Source: three-view drawing plus pictorial views. Frame: mm from the lowest corner of the part. A direction names the side the tool comes from. Coordinates: 2 decimals unless noted, no trailing zeros. Write each loop counter-clockwise with the first axis right and the second up, starting at its lowest first coordinate (ties: lowest second). Pieces come first, ordered by that corner, then holes. Notation, with made-up numbers: (3.25, -17) - (51.25, -17) arc R31 cw to (51.25, 21) - close; hole circle Ø10 at (28.25, -14). An arc over 180 degrees is marked (long way). Answer as a JSON object with one key per item and string values. Group by question number.
Item 1: Section A-A on x = 18. Return loops of the section in (y, z).
Item 2: Section C-C on z = 143. Return loops of the section in (x, y).
Item 3: Set-up query: the marked faces 4, 5 and 6. Return all of +Z, -Z, +X, -X, +Y, -Y with unobstructed straight access to the full face (end or side cutting, diameter ignored); none if empty.
Item 4: Mould query, pull axis Z, two halves, no side actions, for the marked faces 1, 2 and 3. Classes: pulls with the +Z half, pulls with the -Z half, needs draft (parallel to the pull), parting line crosses it, or undercut.
Item 5: First-contact query: pin 1 Ø15 at (y, z) = (128.5, 97) entering from +X; pin 2 Ø17 at (x, z) = (22, 64) entering from +Y; pin 3 Ø23 at (x, z) = (32, 120.5) entering from +Y. Flat tips, straight axial feed; report the tip coordinate or a pass-through.
Item 6: Line query: line 1 along Y through (x, z) = (71.5, 204); line 2 along Y through (x, z) = (33, 120); line 3 along Y through (x, z) = (5.5, 87.5). Output: solid intervals per line, ascending. Write a range as from..to.
Item 7: Section B-B on y = 57. Return loops of the section in (x, z), and give its area (3 significant figures).
Item 8: Section D-D on x = 51. Return loops of the section in (y, z), and give its area (3 significant figures).
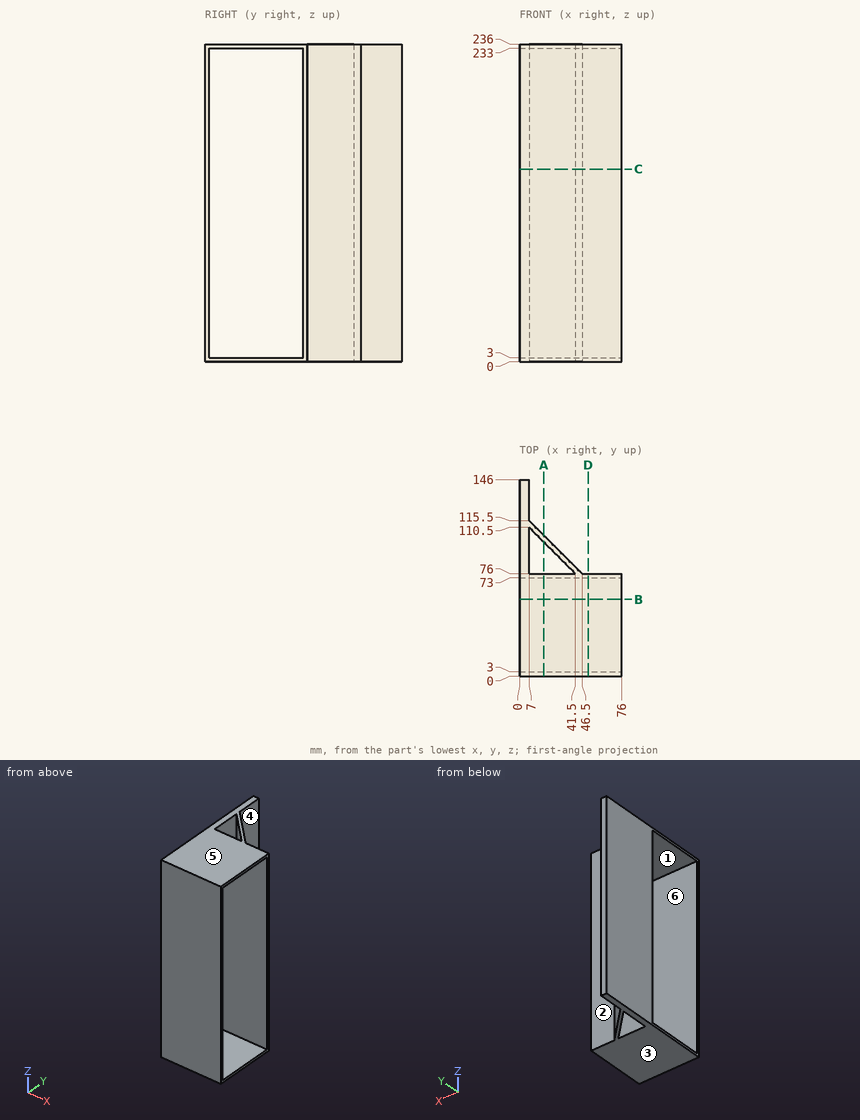
Checks:
{
 "1": {"outline": "(0, 0) - (76, 0) - (76, 236) - (0, 236) - close; (99.5, 0) - (104.5, 0) - (104.5, 236) - (99.5, 236) - close; hole (3, 3) - (73, 3) - (73, 233) - (3, 233) - close"},
 "2": {"outline": "(0, 0) - (76, 0) - (76, 3) - (0, 3) - close; (0, 73) - (76, 73) - (76, 76) - (46.5, 76) - (7, 115.5) - (7, 146) - (0, 146) - close; hole (7, 76) - (41.5, 76) - (7, 110.5) - close"},
 "3": {"face 4": "+Z, -Z, +X, +Y", "face 5": "+Z, +X, -X, +Y, -Y", "face 6": "+X, -X"},
 "4": {"face 1": "undercut", "face 2": "needs draft", "face 3": "pulls with the -Z half"},
 "5": {"pin 1": "x = 7", "pin 2": "y = 109", "pin 3": "y = 102"},
 "6": {"line 1": "0..3, 73..76", "line 2": "0..3, 73..76, 84.5..89.5", "line 3": "0..3, 73..146"},
 "7": {"outline": "(0, 0) - (76, 0) - (76, 3) - (0, 3) - close; (0, 233) - (76, 233) - (76, 236) - (0, 236) - close", "area": "456 mm^2"},
 "8": {"outline": "(0, 0) - (76, 0) - (76, 236) - (0, 236) - close; hole (3, 3) - (73, 3) - (73, 233) - (3, 233) - close", "area": "1,840 mm^2"}
}
